```python
from build123d import *

# Parameters (mm, degrees)
SKETCH1_R           = 5.5
BOSS_EXTRUDE1_DEPTH = 2
SKETCH2_R           = 5
BOSS_EXTRUDE2_DEPTH = 8
SKETCH4_R           = 0.5
BOSS_EXTRUDE3_DEPTH = 10


# Read off the part's stored shape, not the designer's step: Dome1
with BuildPart() as part:
    # Sketch1 → Boss-Extrude1 (new body)
    with BuildSketch(Plane(origin=(0, 0, 0), x_dir=(1, 0, 0), z_dir=(0, 1, 0))):
        with Locations(Location((0, 0, 0), (0, 0, 270))):
            Circle(SKETCH1_R)
    extrude(amount=BOSS_EXTRUDE1_DEPTH)

    # Sketch2 → Boss-Extrude2 (add)
    with BuildSketch(Plane(origin=(0, 2, 0), x_dir=(1, 0, 0), z_dir=(0, 1, 0))):
        with Locations(Location((0, 0, 0), (0, 0, 270))):
            Circle(SKETCH2_R)
    extrude(amount=BOSS_EXTRUDE2_DEPTH)

    # Dome1 outline → Dome1 (revolve)
    with BuildSketch(Plane.XY):
        with BuildLine():
            Line((0, 10), (5, 9.999999995))
            ThreePointArc((5, 9.999999995), (3.535533908, 13.535533904), (0, 15))
            Line((0, 15), (0, 10))
        make_face()
    revolve(axis=Axis((0, 0, 0), (0, 1, 0)))

    # Sketch4 → Boss-Extrude3 (add)
    with BuildSketch(Plane.XZ):
        with Locations(Location((-2, 0, 0), (0, 0, 90))):
            Circle(SKETCH4_R)
        with Locations(Location((2, 0, 0), (0, 0, 90))):
            Circle(SKETCH4_R)
    extrude(amount=BOSS_EXTRUDE3_DEPTH)


solid = part.part
```
Can you work these out from the model? Positions are in its coordinate system, mm. A direction names the side the tool comes from. Coordinates: 2 decimals unless noted, no trailing zeros. Order: outer loops, then holes, each group sorted by start corner. A loop starts at its lowest first (then second) coordinate and runs counter-clockwise, first axis right, second up. Notation, with made-up numbers: (37.5, 32.25) -> (85.5, 32.25) arc R22 cw to (85.5, 38.25) -> close; hole circle Ø2 at (-3, 46.25). An arc over 180 degrees is marked (long way). Write each question's results on one line, items separated by ' | '.
Item 1: I want a section at D-D, the plane x = 4.25. Write out the boundary of the cut face in (y, z).
Results are:
outline: (0, -3.49) -> (2, -3.49) -> (2, -2.63) -> (10, -2.63) arc R2.63 ccw to (10, 2.63) -> (2, 2.63) -> (2, 3.49) -> (0, 3.49) -> close
Item 2: I'm going to push flat-ended pins straight in: pin 1 Ø5.5 at (x, z) = (-1, 2) entering from +Y; pin 2 Ø1 at (x, y) = (0, 6.5) entering from -Z; pin 3 Ø1.5 at (x, z) = (-1, 2.5) entering from -Y; pin 4 Ø2 at (x, z) = (3.5, -1) entering from +Y. Where does each tip first touch, or does it pass through?
Results are:
pin 1: y = 15 | pin 2: z = -5 | pin 3: y = 0 | pin 4: y = 14.25
Item 3: I want a section at B-B, the plane x = 0. Write out the boundary of the cut face in (y, z), then the cut area to 3 significant figures.
Results are:
outline: (0, -5.5) -> (2, -5.5) -> (2, -5) -> (10, -5) arc R5 ccw to (10, 5) -> (2, 5) -> (2, 5.5) -> (0, 5.5) -> close | area: 141 mm²
Item 4: I want a section at C-C, the plane y = 5.75. Write out the boundary of the cut face in (x, z).
Results are:
outline: circle Ø10 at (0, 0)
Item 5: If I drill on line 1 along Y through (x, z) = (-2.25, 4.75); line 2 along X through (y, z) = (5.5, -0.25); line 3 along X through (y, z) = (12.75, -2.75), over which ranges is the centre line in solid material (lowest first)?
Results are:
line 1: 0 to 2 | line 2: -4.99 to 4.99 | line 3: -3.14 to 3.14
Item 6: Which directions (+Z, -Z, +X, -X, +Y, -Y) give clear straight access to the entire face, cutting with the end or side of a thin tool? Please do faces 1 (the face through (-4.9, 2, 1.6)), 2 (the face through (-2, -10, 0)), 3 (the face through (1.504, -4.93, -0.065)).
Results are:
face 1: +Y | face 2: +Z, -Z, +X, -X, -Y | face 3: -Y
Item 7: If we mould it in two halves opening along X, with no side actions, what happens to faces 4 (the face through (-2.496, -4.93, -0.065)), 5 (the face through (2, -10, 0)), 6 (the face through (-5.37, 0.99, -1.19))? For each: +X half, -X half, draft (parallel to the pull), parting line (faces both ways), or undercut.
Results are:
face 4: undercut | face 5: draft | face 6: parting line
Item 8: I want a section at A-A, the plane z = 0. Write out the boundary of the cut face in (x, y).
Results are:
outline: (-5.5, 0) -> (-2.5, 0) -> (-2.5, -10) -> (-1.5, -10) -> (-1.5, 0) -> (1.5, 0) -> (1.5, -10) -> (2.5, -10) -> (2.5, 0) -> (5.5, 0) -> (5.5, 2) -> (5, 2) -> (5, 10) arc R5 ccw to (-5, 10) -> (-5, 2) -> (-5.5, 2) -> close
